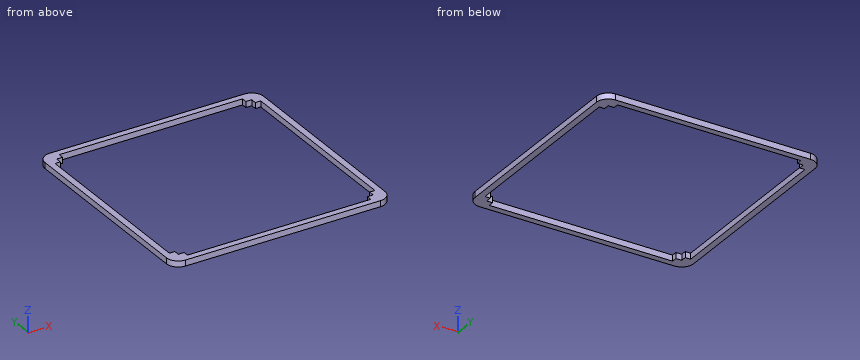
```python
from build123d import *

# Parameters (mm, degrees)
EXTRUDE_1_DEPTH = 3


with BuildPart() as part:
    # 草图1 → 凸台-拉伸1 (new body)
    with BuildSketch(Plane.XY):
        with BuildLine():
            ThreePointArc((-6, 0), (-4.242640687, -4.242640687), (0, -6))
            Line((0, -6), (100, -6))
            ThreePointArc((100, -6), (104.242640687, -4.242640687), (106, 0))
            Line((106, 0), (106, 100))
            ThreePointArc((106, 100), (104.242640687, 104.242640687), (100, 106))
            Line((100, 106), (0, 106))
            ThreePointArc((0, 106), (-4.242640687, 104.242640687), (-6, 100))
            Line((-6, 100), (-6, 0))
        make_face()
        Polygon((97, 0), (97, -2.75), (3, -2.75), (3, 0), (0, 0), (0, 2.885491928), (-2.75, 2.885491928), (-2.75, 3.015491928), (-2.75, 97), (0, 97), (0, 100), (3, 100), (3, 102.75), (97, 102.75), (97, 100), (100, 100), (100, 97), (102.75, 97), (102.75, 3), (100, 3), (100, 0), align=None, mode=Mode.SUBTRACT)
    extrude(amount=EXTRUDE_1_DEPTH)


solid = part.part
```
Geometry check sheet. Reference: the model listing, model coordinates, mm. Round coordinates to 2 decimals unless told otherwise and drop trailing zeros. Write each loop counter-clockwise with the first axis right and the second up, starting at its lowest first coordinate (ties: lowest second). Pieces come first, ordered by that corner, then holes. Notation, with made-up numbers: (58.25, 81) -> (97.25, 81) arc R31 cw to (97.25, 106) -> close; hole circle Ø1 at (-38, -28.75). An arc over 180 degrees is marked (long way). Put each result on its own line as item: value.
1) Cross-section at A-A, the plane y = 8.5. Enter the section's corners in (x, z).
Recorded:
outline: (-6, 0) -> (-2.75, 0) -> (-2.75, 3) -> (-6, 3) -> close; (102.75, 0) -> (106, 0) -> (106, 3) -> (102.75, 3) -> close
2) Thickness scan on probe 1 along X at (y, z) = (66.5, 2.75); probe 2 along Y at (x, z) = (97.5, 1.9). Record the ranges inside material, lowest first. Write a range as from..to.
Recorded:
probe 1: x = -6..-2.75, 102.75..106
probe 2: y = -6..0, 100..106
3) Cross-section at B-B, the plane z = 1.15. Enter the section's corners in (x, y).
Recorded:
outline: (-6, 0) arc R6 ccw to (0, -6) -> (100, -6) arc R6 ccw to (106, 0) -> (106, 100) arc R6 ccw to (100, 106) -> (0, 106) arc R6 ccw to (-6, 100) -> close; hole (-2.75, 2.89) -> (0, 2.89) -> (0, 0) -> (3, 0) -> (3, -2.75) -> (97, -2.75) -> (97, 0) -> (100, 0) -> (100, 3) -> (102.75, 3) -> (102.75, 97) -> (100, 97) -> (100, 100) -> (97, 100) -> (97, 102.75) -> (3, 102.75) -> (3, 100) -> (0, 100) -> (0, 97) -> (-2.75, 97) -> close
4) Depth check by flat-ended pin: P1, Ø0.8, axis at x = 101.5, z = 2, coming from the +Y side; P2, Ø0.8, axis at y = 101, z = 1, coming from the +X side. Enter the tip coordinate at first touch or a pass-through.
Recorded:
P1: stops at y = 105.9
P2: stops at x = 105.97
